The listing builds one solid part. Answer for the finished solid, in the listing's coordinates (mm). A direction names the side the tool comes from. Coordinates: 2 decimals unless noted, no trailing zeros. Write each loop counter-clockwise with the first axis right and the second up, starting at its lowest first coordinate (ties: lowest second). Pieces come first, ordered by that corner, then holes.
from build123d import *

# Parameters (mm, degrees)
BROCA_DE_ROSQUEAR_PARA_TARRAXA_DE_M161_D       = 14
BROCA_DE_ROSQUEAR_PARA_TARRAXA_DE_M161_DEPTH   = 30
BROCA_DE_ROSQUEAR_PARA_TARRAXA_DE_M161_TIP     = 4.206024333
BROCA_DE_ROSQUEAR_PARA_TARRAXA_DE_M161_O_D     = 14
BROCA_DE_ROSQUEAR_PARA_TARRAXA_DE_M161_O_DEPTH = 30
BROCA_DE_ROSQUEAR_PARA_TARRAXA_DE_M161_O_TIP   = 4.206024333
FILETE1_R                                      = 1


with BuildPart() as part:
    # Esboço1 → Revolução1 (revolve)
    with BuildSketch(Plane.XY, mode=Mode.PRIVATE) as revolu_o1_sk:
        Polygon((0, 0), (0, 18), (20, 18), (20, 27), (43, 27), (43, 22.5), (180, 22.5), (180, 18), (200, 18), (200, 0), align=None)
    revolve(revolu_o1_sk.sketch.rotate(Axis((0, 0, 0), (1, 0, 0)), 90), axis=Axis((0, 0, 0), (1, 0, 0)))

    # Broca de rosquear para tarraxa de M161
    with Locations(Plane(origin=(200, 0, 0), x_dir=(0, 0, 1), z_dir=(1, 0, 0))):
        with Locations((0, 0)):
            Hole(BROCA_DE_ROSQUEAR_PARA_TARRAXA_DE_M161_D / 2, depth=BROCA_DE_ROSQUEAR_PARA_TARRAXA_DE_M161_DEPTH)
            with Locations((0, 0, -(BROCA_DE_ROSQUEAR_PARA_TARRAXA_DE_M161_DEPTH + BROCA_DE_ROSQUEAR_PARA_TARRAXA_DE_M161_TIP / 2))):  # 118° drill point
                Cone(0, BROCA_DE_ROSQUEAR_PARA_TARRAXA_DE_M161_D / 2, BROCA_DE_ROSQUEAR_PARA_TARRAXA_DE_M161_TIP, mode=Mode.SUBTRACT)

    # Broca de rosquear para tarraxa de M161 o
    with Locations(Plane(origin=(0, 0, 0), x_dir=(0, 0, -1), z_dir=(-1, 0, 0))):
        with Locations((0, 0)):
            Hole(BROCA_DE_ROSQUEAR_PARA_TARRAXA_DE_M161_O_D / 2, depth=BROCA_DE_ROSQUEAR_PARA_TARRAXA_DE_M161_O_DEPTH)
            with Locations((0, 0, -(BROCA_DE_ROSQUEAR_PARA_TARRAXA_DE_M161_O_DEPTH + BROCA_DE_ROSQUEAR_PARA_TARRAXA_DE_M161_O_TIP / 2))):  # 118° drill point
                Cone(0, BROCA_DE_ROSQUEAR_PARA_TARRAXA_DE_M161_O_D / 2, BROCA_DE_ROSQUEAR_PARA_TARRAXA_DE_M161_O_TIP, mode=Mode.SUBTRACT)

    # Filete1
    filete1_edges = [part.edges().sort_by_distance(p)[0] for p in [
        (20, 0, -18),
        (180, 0, -18),
        (43, 0, -22.5),
    ]]
    fillet(filete1_edges, radius=FILETE1_R)


solid = part.part
1. Flat-ended cylindrical pins translate along their axes: P1, Ø18, axis at y = 0, z = 0, coming from the -X side; P2, Ø4, axis at x = 115, y = 18.5, coming from the +Z side; P3, Ø1.5, axis at x = 157.5, y = -3.5, coming from the +Z side; P4, Ø1, axis at x = 147.5, y = 8, coming from the -Z side. Find the tip coordinate at first contact, or state that the pin passes through.
Results found:
P1: stops at x = 0
P2: stops at z = 15.3
P3: stops at z = 22.33
P4: stops at z = -21.21
2. Section B-B on x = 160.5 is taken. Give the vertices of the cut face in (y, z).
Results found:
outline: circle Ø45 at (0, 0)
3. A tool of negligible diameter and unlimited length cuts with its end or side. For faces 1 (the cylindrical face through (31.66, 26.36, -5.85)), 2 (the cylindrical face through (190.633, -12.165, -13.267)), 3 (the cylindrical face through (9.633, -12.165, -13.267)), from which of +Z, -Z, +X, -X, +Y, -Y can it reach the whole face along a straight path? Write none if from no direction.
Results found:
face 1: +X, -X
face 2: +X
face 3: -X
4. Section A-A on x = 39 is taken. Give the vertices of the cut face in (y, z).
Results found:
outline: circle Ø54 at (0, 0)
5. Find the intervals of material crossed by L1, parallel to Y at x = 12.75, z = 0; L2, parallel to Y at x = 23, z = 0; L3, parallel to X at y = 9.5, z = -19.5, in increasing order.
Results found:
L1: y = -18 to -7, 7 to 18
L2: y = -27 to -7, 7 to 27
L3: x = 20 to 180
